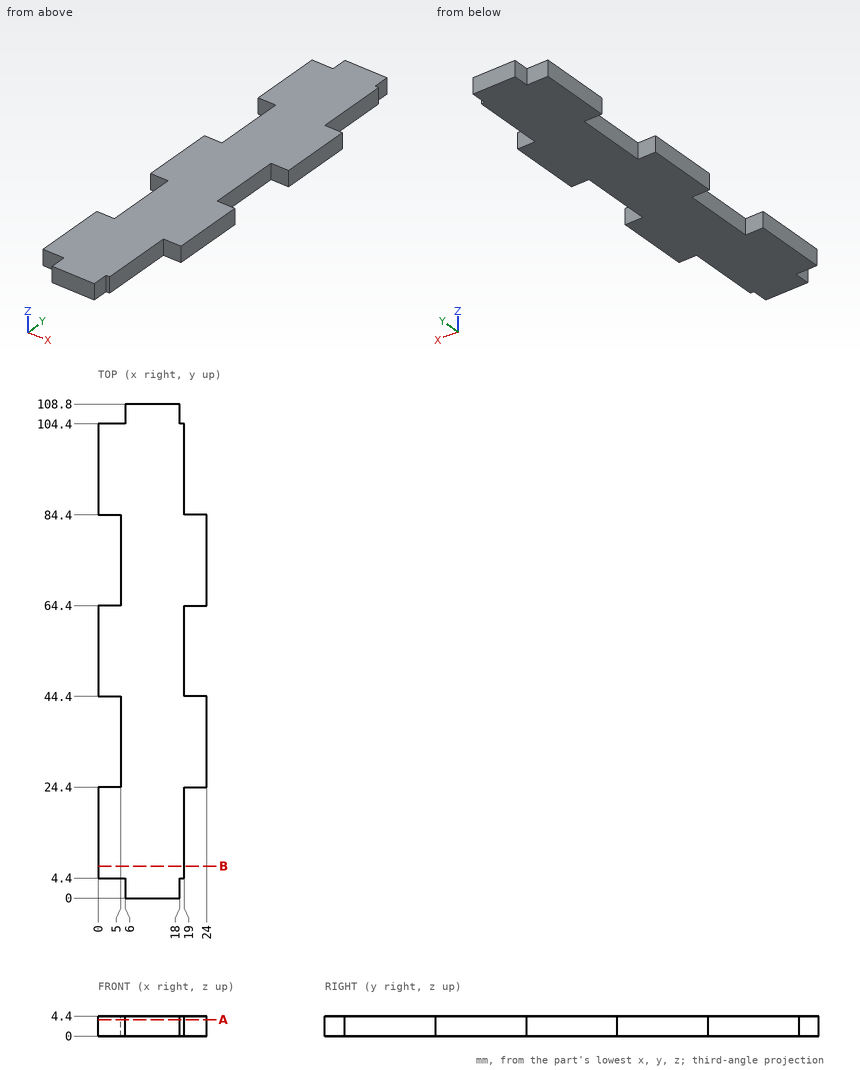
Can you work these out from the drawing? Everything is in mm from the part's minimum corner. Coordinates: 2 decimals unless noted, no trailing zeros. Loops run counter-clockwise (first coordinate to the right, second up) from the corner with the lowest first, then second, coordinate; pieces in that order, holes last. Notation, with made-up numbers: (36, 66) -> (86, 66) arc R17 cw to (86, 70) -> close; hole circle Ø1 at (35, -39). An arc over 180 degrees is marked (long way). Return JSON: item names as keys, results as strings.
1) Will these pins go through, and if not, where does the flat tip stop? pin 1 (1.3 mm diameter, centred on y = 2.5, z = 1, fed in from +X); pin 2 (1.5 mm diameter, centred on x = 20, z = 3, fed in from -Y); pin 3 (0.5 mm diameter, centred on x = 18.5, z = 2, fed in from -Y).
Results below:
{"pin 1": "x = 18", "pin 2": "y = 24.4", "pin 3": "y = 4.4"}
2) I need wall thicknesses on line 1 (Y direction, x = 2.25, z = 0.5); line 2 (X direction, y = 71.5, z = 2.3); line 3 (X direction, y = 8, z = 2.35). Which ranges of each line are inside material? Lowest first, please. Write a range as from..to.
Results below:
{"line 1": "4.4..24.4, 44.4..64.4, 84.4..104.4", "line 2": "5..24", "line 3": "0..19"}
3) If we section it at A-A, the plane z = 3.6: Write out the boundary of the cut face in (x, y).
Results below:
{"outline": "(0, 4.4) -> (6, 4.4) -> (6, 0) -> (18, 0) -> (18, 4.4) -> (19, 4.4) -> (19, 24.4) -> (24, 24.4) -> (24, 44.4) -> (19, 44.4) -> (19, 64.4) -> (24, 64.4) -> (24, 84.4) -> (19, 84.4) -> (19, 104.4) -> (18, 104.4) -> (18, 108.8) -> (6, 108.8) -> (6, 104.4) -> (0, 104.4) -> (0, 84.4) -> (5, 84.4) -> (5, 64.4) -> (0, 64.4) -> (0, 44.4) -> (5, 44.4) -> (5, 24.4) -> (0, 24.4) -> close"}
4) If we section it at B-B, the plane y = 7: Write out the boundary of the cut face in (x, z).
Results below:
{"outline": "(0, 0) -> (19, 0) -> (19, 4.4) -> (0, 4.4) -> close"}
